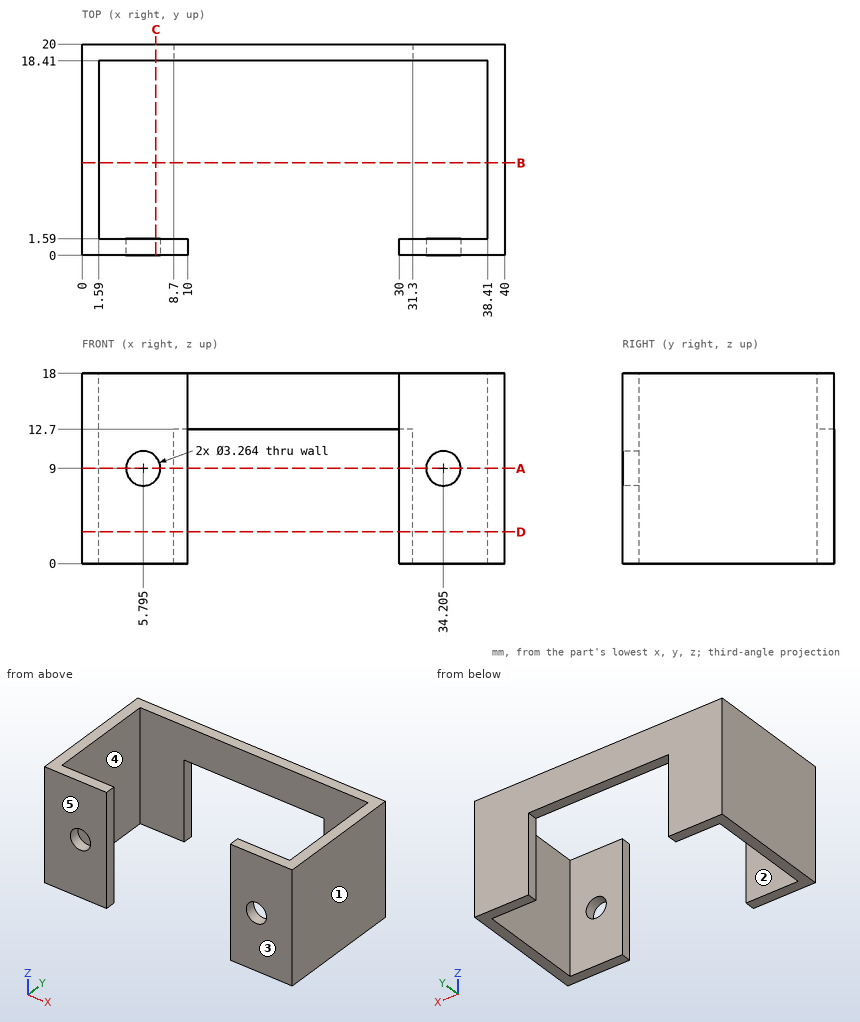
Verification items for this drawing (mm, ordinates from the low corner). A direction names the side the tool comes from. Give positions to 0.01 mm unless a question says otherwise; leave off trailing zeros. Loops run counter-clockwise (first coordinate to the right, second up) from the corner with the lowest first, then second, coordinate; pieces in that order, holes last. Notation, with made-up numbers: (16.5, 87.25) - (46.5, 87.25) arc R9 ccw to (46.5, 103.25) - close; hole circle Ø2 at (-31.75, 47.5). An arc over 180 degrees is marked (long way). Write item = value, one per line. Start each with the question number.
Q1. Thickness scan on line 1 (X direction, y = 0.85, z = 9); line 2 (X direction, y = 3.5, z = 3.75); line 3 (Y direction, x = 4, z = 5.5). Record the ranges inside material, lowest first.
Q2. Cross-section at A-A, the plane z = 9. Enter the section's corners in (x, y).
Q3. Cross-section at B-B, the plane y = 8.75. Enter the section's corners in (x, z).
Q4. Tool access check on the marked faces 4 and 5. Record the directions out of +Z, -Z, +X, -X, +Y, -Y that give a thin tool (end or side, any length) a straight path to the whole face; none if there is none.
Q5. Mould release check, pull along X, two halves, no side actions. Record for the marked faces 1, 2 and 3: released by +X, released by -X, zero draft, split by the parting line, or undercut.
Q6. Cross-section at D-D, the plane z = 3. Enter the section's corners in (x, y), and give its area (3 significant figures).
Q7. Cross-section at C-C, the plane x = 7. Enter the section's corners in (y, z).
Q8. Depth check by flat-ended pin: P1, Ø1.5, axis at x = 24.5, z = 10, coming from the +Y side; P2, Ø1.5, axis at x = 30, z = 7, coming from the +Y side; P3, Ø0.5, axis at x = 23.5, y = 19, coming from the -Z side; P4, Ø3, axis at x = 34.205, z = 9, coming from the -Y side. Enter the tip coordinate at first touch or a pass-through.
Answer key:
q1.line_1 = 0 to 4.16, 7.43 to 10, 30 to 32.57, 35.84 to 40
q1.line_2 = 0 to 1.59, 38.41 to 40
q1.line_3 = 0 to 1.59, 18.41 to 20
q2.outline = (0, 0) - (4.16, 0) - (4.16, 1.59) - (1.59, 1.59) - (1.59, 18.41) - (8.7, 18.41) - (8.7, 20) - (0, 20) - close; (7.43, 0) - (10, 0) - (10, 1.59) - (7.43, 1.59) - close; (30, 0) - (32.57, 0) - (32.57, 1.59) - (30, 1.59) - close; (31.3, 18.41) - (38.41, 18.41) - (38.41, 1.59) - (35.84, 1.59) - (35.84, 0) - (40, 0) - (40, 20) - (31.3, 20) - close
q3.outline = (0, 0) - (1.59, 0) - (1.59, 18) - (0, 18) - close; (38.41, 0) - (40, 0) - (40, 18) - (38.41, 18) - close
q4.face_4 = +Z, -Z
q4.face_5 = +Z, -Z, +X, -X, -Y
q5.face_1 = released by +X
q5.face_2 = undercut
q5.face_3 = zero draft
q6.outline = (0, 0) - (10, 0) - (10, 1.59) - (1.59, 1.59) - (1.59, 18.41) - (8.7, 18.41) - (8.7, 20) - (0, 20) - close; (30, 0) - (40, 0) - (40, 20) - (31.3, 20) - (31.3, 18.41) - (38.41, 18.41) - (38.41, 1.59) - (30, 1.59) - close
q6.area = 113 mm^2
q7.outline = (0, 0) - (1.59, 0) - (1.59, 7.9) - (0, 7.9) - close; (0, 10.1) - (1.59, 10.1) - (1.59, 18) - (0, 18) - close; (18.41, 0) - (20, 0) - (20, 18) - (18.41, 18) - close
q8.P1 = through
q8.P2 = 1.59
q8.P3 = 12.7
q8.P4 = 18.41
